from build123d import *

# Parameters (mm, degrees)
F0_W     = 1500
F0_H     = 1500
F1_DEPTH = 25
F2_SIZE  = 50
F3_W     = 1200
F3_H     = 378
F4_DEPTH = 960
F6_D     = 100
F8_DEPTH = 532.28619
F10_D    = 30


with BuildPart() as f1:
    # F0 (on Top) → F1 (new body)
    with BuildSketch(Plane.XY):
        with Locations((-638.344221, 641.208582)):
            Rectangle(F0_W, F0_H)
    extrude(amount=F1_DEPTH)

    # F2
    f2_edges = [f1.edges().sort_by_distance(p)[0] for p in [
        (-1388.344221, -108.791418, 12.5),
        (111.655779, -108.791418, 12.5),
        (111.655779, 1391.208582, 12.5),
        (-1388.344221, 1391.208582, 12.5),
    ]]
    chamfer(f2_edges, length=F2_SIZE)

    # F3 (on face) → F4 (join)
    with BuildSketch(Plane.XY.offset(25)):
        with Locations((-638.344221, 641.208582)):
            Rectangle(F3_W, F3_H)
    extrude(amount=F4_DEPTH)

    # F6 (through all)
    with Locations(Plane.XZ.offset(-452.208582)):
        with Locations((-638.344221, 885)):
            Hole(F6_D / 2)

    # F7 (on face) → F8 (cut)
    with BuildSketch(Plane.XZ.offset(-452.208582)):
        with BuildLine():
            Line((-1238.344221, 985), (-1238.344221, 225))
            Line((-1238.344221, 225), (-719.413216, 943.547571))
            ThreePointArc((-719.413216, 943.547571), (-683.870273, 974.035827), (-638.344221, 985))
            Line((-638.344221, 985), (-1238.344221, 985))
        make_face()
        with BuildLine():
            Line((-38.344221, 985), (-638.344221, 985))
            ThreePointArc((-638.344221, 985), (-592.818168, 974.035827), (-557.275226, 943.547571))
            Line((-557.275226, 943.547571), (-38.344221, 225))
            Line((-38.344221, 225), (-38.344221, 985))
        make_face()
    extrude(amount=-F8_DEPTH, mode=Mode.SUBTRACT)

    # F10 (through all)
    with Locations(Plane(origin=(0, 0, 0), x_dir=(1, 0, 0), z_dir=(0, 0, -1))):
        with Locations((-1282.406457, -1291.193252), (-1132.406457, -1291.193252), (-1132.406457, -1141.193252), (-1282.406457, -1141.193252), (-1288.344221, -141.208582), (-1138.344221, -141.208582), (-1138.344221, 8.791418), (-1288.344221, 8.791418), (-138.344221, 8.791418), (11.655779, 8.791418), (11.655779, -141.208582), (-138.344221, -141.208582), (-132.406457, -1141.193252), (17.593543, -1141.193252), (17.593543, -1291.193252), (-132.406457, -1291.193252)):
            Hole(F10_D / 2)


solid = f1.part
Verification items for the finished model (mm, model axes). A direction names the side the tool comes from. Coordinates: 2 decimals unless noted, no trailing zeros. Write each loop counter-clockwise with the first axis right and the second up, starting at its lowest first coordinate (ties: lowest second). Pieces come first, ordered by that corner, then holes. Notation, with made-up numbers: M -39.5,10 L 13.5,10 A33 cw 13.5,46 Z; hole C 73,65.25 d1. An arc over 180 degrees is marked long. One line per question, with ' | ' between items.
1) Release check for a two-part mould opening along Z. For faces 1 (the face through (-301.44, 638.56, 589.3)), 2 (the face through (-665.224, 643.855, 927.16)), 3 (the face through (-647, 452.209, 392)) record: +Z half, -Z half, draft (parallel to the pull), parting line (faces both ways), or undercut.
Solutions:
face 1: +Z half | face 2: undercut | face 3: draft
2) Sectioned sample at D-D on y = 45.5. Record the cut outline in (x, z).
Solutions:
outline: M -1388.34,0 L 111.66,0 L 111.66,25 L -1388.34,25 Z
3) Depth check by flat-ended pin: pin 1 Ø1 at (x, y) = (-1004.5, 912.5) entering from -Z; pin 2 Ø3 at (x, z) = (-989, 288) entering from -Y; pin 3 Ø6 at (x, z) = (-773, 754.5) entering from +Y; pin 4 Ø10 at (x, y) = (-91, 262.5) entering from +Z. Enter the tip coordinate at first touch or a pass-through.
Solutions:
pin 1: z = 0 | pin 2: y = 452.21 | pin 3: y = 830.21 | pin 4: z = 25
4) Access from +Z, -Z, +X, -X, +Y, -Y to the whole of each face (thin tool, end or side, straight path). Record for faces 4 (the face through (-647, 830.209, 392)), 5 (the face through (-1238.344, 639, 124)), 6 (the face through (-38.344, 639, 124)).
Solutions:
face 4: +Z, +X, -X, +Y | face 5: +Z, -X, +Y, -Y | face 6: +Z, +X, +Y, -Y
5) Material ranges on L1, parallel to Z at x = -122.5, y = 310; L2, parallel to Y at x = -614.5, z = 478; L3, parallel to X at y = 682, z = 162.5, recorded low to high.
Solutions:
L1: 0 to 25 | L2: 452.21 to 830.21 | L3: -1238.34 to -38.34
6) Sectioned sample at C-C on x = -793. Record the cut outline in (y, z), then the cut area to 3 significant figures.
Solutions:
outline: M -108.79,0 L 1391.21,0 L 1391.21,25 L 830.21,25 L 830.21,841.65 L 452.21,841.65 L 452.21,25 L -108.79,25 Z | area: 346,000 mm^2
7) Sectioned sample at A-A on y = 529. Record the cut outline in (x, z).
Solutions:
outline: M -1388.34,0 L 111.66,0 L 111.66,25 L -38.34,25 L -38.34,225 L -557.28,943.55 A100 ccw -638.34,985 A100 ccw -719.41,943.55 L -1238.34,225 L -1238.34,25 L -1388.34,25 Z; hole C -638.34,885 d100
8) Sectioned sample at B-B on z = 885. Record the cut outline in (x, y).
Solutions:
outline: M -761.7,452.21 L -688.34,452.21 L -688.34,830.21 L -761.7,830.21 Z; M -588.34,452.21 L -514.99,452.21 L -514.99,830.21 L -588.34,830.21 Z
